Autodesk Inventor part; units mm, degrees
ref_plane "YZ Plane" through (0, 0, 0) normal (1, 0, 0) x (0, 1, 0)
ref_plane "XZ Plane" through (0, 0, 0) normal (0, 1, 0) x (-1, 0, 0)
ref_plane "XY Plane" through (0, 0, 0) normal (0, 0, 1) x (1, 0, 0)
sketch "Sketch1" plane through (0, 0, 0) normal (0, 0, 1) x (1, 0, 0)
  line L0 (-32.7, -6.0134) -> (-32.7, 6.0134)
  arc A0 (-32.6116, 8.9958) -> (-32.7, 6.0134) centre (-32.5, 7.5) ccw
  arc A1 (-20, 20.2) -> (-32.6116, 8.9958) centre (-20, 7.5) ccw
  line L1 (-20, 20.2) -> (-16.9142, 20.2)
  arc A2 (-14.0858, 20.2) -> (-16.9142, 20.2) centre (-15.5, 19.7) ccw
  line L2 (-14.0858, 20.2) -> (14.0858, 20.2)
  arc A3 (16.9142, 20.2) -> (14.0858, 20.2) centre (15.5, 19.7) ccw
  line L3 (16.9142, 20.2) -> (20, 20.2)
  arc A4 (32.6116, 8.9958) -> (20, 20.2) centre (20, 7.5) ccw
  arc A5 (32.7, 6.0134) -> (32.6116, 8.9958) centre (32.5, 7.5) ccw
  line L4 (32.7, 6.0134) -> (32.7, -6.0134)
  arc A6 (32.6116, -8.9958) -> (32.7, -6.0134) centre (32.5, -7.5) ccw
  arc A7 (20, -20.2) -> (32.6116, -8.9958) centre (20, -7.5) ccw
  line L5 (20, -20.2) -> (16.9142, -20.2)
  arc A8 (14.0858, -20.2) -> (16.9142, -20.2) centre (15.5, -19.7) ccw
  line L6 (14.0858, -20.2) -> (-14.0858, -20.2)
  arc A9 (-16.9142, -20.2) -> (-14.0858, -20.2) centre (-15.5, -19.7) ccw
  line L7 (-16.9142, -20.2) -> (-20, -20.2)
  arc A10 (-32.6116, -8.9958) -> (-20, -20.2) centre (-20, -7.5) ccw
  arc A11 (-32.7, -6.0134) -> (-32.6116, -8.9958) centre (-32.5, -7.5) ccw
  arc A12 (34.6474, -8.7801) -> (34.7032, -6.3185) centre (32.5, -7.5) ccw
  line L8 (34.7032, -6.3185) -> (34.7032, 6.3185)
  arc A13 (34.7032, 6.3185) -> (34.6474, 8.7801) centre (32.5, 7.5) ccw
  arc A14 (34.6474, 8.7801) -> (20, 22.2032) centre (20, 7.5) ccw
  line L9 (20, 22.2032) -> (-20, 22.2032)
  arc A15 (-20, 22.2032) -> (-34.6474, 8.7801) centre (-20, 7.5) ccw
  arc A16 (-34.6474, 8.7801) -> (-34.7032, 6.3185) centre (-32.5, 7.5) ccw
  line L10 (-34.7032, 6.3185) -> (-34.7032, -6.3185)
  arc A17 (-34.7032, -6.3185) -> (-34.6474, -8.7801) centre (-32.5, -7.5) ccw
  arc A18 (-34.6474, -8.7801) -> (-20, -22.2032) centre (-20, -7.5) ccw
  line L11 (-20, -22.2032) -> (20, -22.2032)
  arc A19 (20, -22.2032) -> (34.6474, -8.7801) centre (20, -7.5) ccw
  arc A20 (-31.6356, 8.7259) -> (-32.6116, 8.9958) centre (-32.5, 7.5) ccw
  arc A21 (-20, 19.2) -> (-31.6356, 8.7259) centre (-20, 7.5) ccw
  line L12 (-16.9142, 19.2) -> (-20, 19.2)
  arc A22 (-16.9142, 20.2) -> (-16.9142, 19.2) centre (-15.5, 19.7) ccw
  line L13 (-20, 20.2) -> (-16.9142, 20.2)
  arc A23 (-20, 20.2) -> (-32.6116, 8.9958) centre (-20, 7.5) ccw
  arc A24 (-32.7, 6.0134) -> (-31.7, 6.2311) centre (-32.5, 7.5) ccw
  line L14 (-32.7, -6.0134) -> (-32.7, 6.0134)
  arc A25 (-31.7, -6.2311) -> (-32.7, -6.0134) centre (-32.5, -7.5) ccw
  line L15 (-31.7, 6.2311) -> (-31.7, -6.2311)
  line L16 (-31.7, 6.2311) -> (-31.7, -6.2311)
  arc A26 (-31.6356, -8.7259) -> (-31.7, -6.2311) centre (-32.5, -7.5) ccw
  arc A27 (-31.6356, -8.7259) -> (-20, -19.2) centre (-20, -7.5) ccw
  line L17 (-20, -19.2) -> (-16.9142, -19.2)
  arc A28 (-14.0858, -19.2) -> (-16.9142, -19.2) centre (-15.5, -19.7) ccw
  line L18 (-14.0858, -19.2) -> (14.0858, -19.2)
  arc A29 (16.9142, -19.2) -> (14.0858, -19.2) centre (15.5, -19.7) ccw
  line L19 (16.9142, -19.2) -> (20, -19.2)
  arc A30 (20, -19.2) -> (31.6356, -8.7259) centre (20, -7.5) ccw
  arc A31 (31.7, -6.2311) -> (31.6356, -8.7259) centre (32.5, -7.5) ccw
  line L20 (31.7, -6.2311) -> (31.7, 6.2311)
  arc A32 (31.6356, 8.7259) -> (31.7, 6.2311) centre (32.5, 7.5) ccw
  arc A33 (31.6356, 8.7259) -> (20, 19.2) centre (20, 7.5) ccw
  line L21 (20, 19.2) -> (16.9142, 19.2)
  arc A34 (14.0858, 19.2) -> (16.9142, 19.2) centre (15.5, 19.7) ccw
  line L22 (14.0858, 19.2) -> (-14.0858, 19.2)
  arc A35 (-16.9142, 19.2) -> (-14.0858, 19.2) centre (-15.5, 19.7) ccw
  line L23 (-16.9142, 19.2) -> (-20, 19.2)
  arc A36 (-20, 19.2) -> (-31.6356, 8.7259) centre (-20, 7.5) ccw
  arc A37 (-31.7, 6.2311) -> (-31.6356, 8.7259) centre (-32.5, 7.5) ccw
  line L24 (-30.1616, -8.3842) -> (-30.2, -6.5202)
  line L25 (-30.2, -6.5202) -> (-30.2, 6.5202)
  line L26 (-30.2, 6.5202) -> (-30.1616, 8.3842)
  arc A38 (-20, 17.7) -> (-30.1616, 8.3842) centre (-20, 7.5) ccw
  line L27 (-20, 17.7) -> (20, 17.7)
  arc A39 (30.1616, 8.3842) -> (20, 17.7) centre (20, 7.5) ccw
  line L28 (30.1616, 8.3842) -> (30.2, 6.5202)
  line L29 (30.2, 6.5202) -> (30.2, -6.5202)
  line L30 (30.2, -6.5202) -> (30.1616, -8.3842)
  arc A40 (20, -17.7) -> (30.1616, -8.3842) centre (20, -7.5) ccw
  line L31 (20, -17.7) -> (-20, -17.7)
  arc A41 (-30.1616, -8.3842) -> (-20, -17.7) centre (-20, -7.5) ccw
  arc A42 (-14.0858, -20.2) -> (-14.0858, -19.2) centre (-15.5, -19.7) ccw
  line L32 (14.0858, -20.2) -> (-14.0858, -20.2)
  arc A43 (14.0858, -19.2) -> (14.0858, -20.2) centre (15.5, -19.7) ccw
  line L33 (-14.0858, -19.2) -> (14.0858, -19.2)
  arc A44 (-16.9142, -19.2) -> (-16.9142, -20.2) centre (-15.5, -19.7) ccw
  line L34 (-20, -19.2) -> (-16.9142, -19.2)
  arc A45 (-31.6356, -8.7259) -> (-20, -19.2) centre (-20, -7.5) ccw
  arc A46 (-32.6116, -8.9958) -> (-31.6356, -8.7259) centre (-32.5, -7.5) ccw
  arc A47 (-32.6116, -8.9958) -> (-20, -20.2) centre (-20, -7.5) ccw
  line L35 (-16.9142, -20.2) -> (-20, -20.2)
  arc A48 (31.6356, -8.7259) -> (32.6116, -8.9958) centre (32.5, -7.5) ccw
  arc A49 (20, -19.2) -> (31.6356, -8.7259) centre (20, -7.5) ccw
  line L36 (16.9142, -19.2) -> (20, -19.2)
  arc A50 (16.9142, -20.2) -> (16.9142, -19.2) centre (15.5, -19.7) ccw
  line L37 (20, -20.2) -> (16.9142, -20.2)
  arc A51 (20, -20.2) -> (32.6116, -8.9958) centre (20, -7.5) ccw
  arc A52 (-14.0858, -20.2) -> (-14.0858, -19.2) centre (-15.5, -19.7) ccw
  line L38 (14.0858, -20.2) -> (-14.0858, -20.2)
  arc A53 (14.0858, -19.2) -> (14.0858, -20.2) centre (15.5, -19.7) ccw
  line L39 (-14.0858, -19.2) -> (14.0858, -19.2)
  arc A54 (32.7, -6.0134) -> (31.7, -6.2311) centre (32.5, -7.5) ccw
  line L40 (32.7, 6.0134) -> (32.7, -6.0134)
  arc A55 (31.7, 6.2311) -> (32.7, 6.0134) centre (32.5, 7.5) ccw
  line L41 (31.7, -6.2311) -> (31.7, 6.2311)
  arc A56 (16.9142, 19.2) -> (16.9142, 20.2) centre (15.5, 19.7) ccw
  line L42 (20, 19.2) -> (16.9142, 19.2)
  arc A57 (31.6356, 8.7259) -> (20, 19.2) centre (20, 7.5) ccw
  arc A58 (32.6116, 8.9958) -> (31.6356, 8.7259) centre (32.5, 7.5) ccw
  arc A59 (32.6116, 8.9958) -> (20, 20.2) centre (20, 7.5) ccw
  line L43 (16.9142, 20.2) -> (20, 20.2)
  arc A60 (14.0858, 20.2) -> (14.0858, 19.2) centre (15.5, 19.7) ccw
  line L44 (-14.0858, 20.2) -> (14.0858, 20.2)
  arc A61 (-14.0858, 19.2) -> (-14.0858, 20.2) centre (-15.5, 19.7) ccw
  line L45 (14.0858, 19.2) -> (-14.0858, 19.2)
  point P0 (0, 0)
extrude "Extrusion1" add sketch "Sketch1" along normal blind 2.5 contours L0 A24 L15 A25 | A46 A27 L17 A44 L7 A10 | L15 A37 A21 L12 A35 L22 A34 L21 A33 A32 L20 A31 A30 L19 A29 L18 A28 L17 A27 A26 | A1 L1 A22 L12 A21 A20 | A42 L18 A43 L6 | L2 A60 L22 A61 | A50 L19 A30 A48 A7 L5 | L3 A4 A58 A33 L21 A56 | A54 L20 A55 L4 | A19 L11 A18 A17 L10 A16 A15 L9 A14 A13 L8 A12 | L24 L25 L26 A38 L27 A39 L28 L29 L30 A40 L31 A41
properties part number "front_acryl"
Model file for the job. Use its own axes, mm. A direction names the side the tool comes from. Coordinates: 2 decimals unless noted, no trailing zeros. Write each loop counter-clockwise with the first axis right and the second up, starting at its lowest first coordinate (ties: lowest second). Pieces come first, ordered by that corner, then holes. Notation, with made-up numbers: (24.5, 34.5) - (28.5, 34.5) arc R16 ccw to (28.5, 57.5) - close; hole circle Ø5 at (-38, -17). An arc over 180 degrees is marked (long way). One line per item, written item: value. Start each with the question number.
1. Slice it at B-B (z = 0.6). Count the separate pieces of the cut face and the enclosed holes in it, plus the area to 3 significant figures.
2. Tool access for faces 1 (the cylindrical face through (-29.821, -18.442, 1.232)), 2 (the cylindrical face through (-34, 7.5, 1.2)): list every direction of +Z, -Z, +X, -X, +Y, -Y with a clear straight run to the whole face (end or side of a thin tool).
3. Slice it at C-C (x = -16). Write the cut outline in (y, z), plus the area to 3 significant figures.
4. Flat gauge pins, fed straight in: pin 1 (1 mm diameter, centred on y = -1, z = 2, fed in from -X); pin 2 (3.5 mm diameter, centred on x = 15.5, y = -19.7, fed in from -Z). Where does each tip first touch, or does it go through?
5. Probe line 1 (Y direction, x = -15.5, z = 1.6); line 2 (X direction, y = 7.5, z = 0.75); line 3 (X direction, y = 8, z = 2.3). List the from-to ranges inside material, lowest first. Write a range as from..to.
6. Slice it at A-A (x = 15.5). Write the cut outline in (y, z), plus the area to 3 significant figures.
7. Mould opens along X. For faces 3 (the cylindrical face through (29.821, 18.442, 1.232)), 4 (the flat face through (0, 0, 2.5)), 5 (the cylindrical face through (34, -7.5, 1.2)) say: released by +X, released by -X, zero draft, split by the parting line, or undercut.
Answers below:
1. separate pieces: 1
1. enclosed holes: 8
1. area: 2,840 mm^2
2. face 1: +Z, -Z, -X, -Y
2. face 2: +Z, -Z
3. outline: (-22.2, 0) - (-21.11, 0) - (-21.11, 2.5) - (-22.2, 2.5) - close; (-18.29, 0) - (18.29, 0) - (18.29, 2.5) - (-18.29, 2.5) - close; (21.11, 0) - (22.2, 0) - (22.2, 2.5) - (21.11, 2.5) - close
3. area: 96.9 mm^2
4. pin 1: stops at x = -34.7
4. pin 2: stops at z = 0
5. line 1: y = -22.2..-21.2, -18.2..18.2, 21.2..22.2
5. line 2: x = -35..-34, -31..31, 34..35
5. line 3: x = -34.95..-33.91, -31.09..31.09, 33.91..34.95
6. outline: (-22.2, 0) - (-21.2, 0) - (-21.2, 2.5) - (-22.2, 2.5) - close; (-18.2, 0) - (18.2, 0) - (18.2, 2.5) - (-18.2, 2.5) - close; (21.2, 0) - (22.2, 0) - (22.2, 2.5) - (21.2, 2.5) - close
6. area: 96.0 mm^2
7. face 3: released by +X
7. face 4: zero draft
7. face 5: undercut
